from build123d import *

# Parameters (mm, degrees)
SKETCH1_W      = 31.75
SKETCH1_H      = 44.45
EXTRUDE1_DEPTH = 380


with BuildPart() as part:
    # Sketch1 → Extrude1 (new body)
    with BuildSketch(Plane(origin=(0, 0, 0), x_dir=(0, 0, -1), z_dir=(1, 0, 0))):
        with BuildLine():
            Line((-15.875, 25.4), (15.875, 25.4))
            ThreePointArc((15.875, 25.4), (18.12006403, 24.47006403), (19.05, 22.225))
            Line((19.05, 22.225), (19.05, -22.225))
            ThreePointArc((19.05, -22.225), (18.12006403, -24.47006403), (15.875, -25.4))
            Line((15.875, -25.4), (-15.875, -25.4))
            ThreePointArc((-15.875, -25.4), (-18.12006403, -24.47006403), (-19.05, -22.225))
            Line((-19.05, -22.225), (-19.05, 22.225))
            ThreePointArc((-19.05, 22.225), (-18.12006403, 24.47006403), (-15.875, 25.4))
        make_face()
        Rectangle(SKETCH1_W, SKETCH1_H, mode=Mode.SUBTRACT)
    extrude(amount=EXTRUDE1_DEPTH)


solid = part.part
Part model, mm, in its own coordinate system. A direction names the side the tool comes from. Round coordinates to 2 decimals unless told otherwise and drop trailing zeros. Loops run counter-clockwise (first coordinate to the right, second up) from the corner with the lowest first, then second, coordinate; pieces in that order, holes last. Notation, with made-up numbers: (0.25, 53) - (34.25, 53) arc R26 cw to (34.25, 68) - close; hole circle Ø4 at (77, 70.5). An arc over 180 degrees is marked (long way). Answer as a JSON object with one key per item and string values.
Item 1: Tool access for faces 1 (the face through (187, 0, -15.875)), 2 (the face through (187, 25.4, 0)): list every direction of +Z, -Z, +X, -X, +Y, -Y with a clear straight run to the whole face (end or side of a thin tool).
Output:
{"face 1": "+X, -X", "face 2": "+Z, -Z, +X, -X, +Y"}
Item 2: Band-saw the part on C-C on x = 212.5. List the corners of the cut face in (y, z) (3 decimals).
Output:
{"outline": "(-25.4, -15.875) arc R3.175 ccw to (-22.225, -19.05) - (22.225, -19.05) arc R3.175 ccw to (25.4, -15.875) - (25.4, 15.875) arc R3.175 ccw to (22.225, 19.05) - (-22.225, 19.05) arc R3.175 ccw to (-25.4, 15.875) - close; hole (-22.225, -15.875) - (22.225, -15.875) - (22.225, 15.875) - (-22.225, 15.875) - close"}
Item 3: Pull direction Z, two halves, no side cores. Call faces 3 (the face through (187, -25.4, 0)), 4 (the face through (187, 0, 19.05)), 5 (the face through (187, 22.225, 0)): pulls with the +Z half, pulls with the -Z half, needs draft (parallel to the pull), parting line crosses it, or undercut.
Output:
{"face 3": "needs draft", "face 4": "pulls with the +Z half", "face 5": "undercut"}
Item 4: Band-saw the part on A-A on z = -4. List the corners of the cut face in (x, y) (3 decimals).
Output:
{"outline": "(0, -25.4) - (380, -25.4) - (380, -22.225) - (0, -22.225) - close; (0, 22.225) - (380, 22.225) - (380, 25.4) - (0, 25.4) - close"}
Item 5: Band-saw the part on B-B on y = 16. List the corners of the cut face in (x, z) (3 decimals).
Output:
{"outline": "(0, -19.05) - (380, -19.05) - (380, -15.875) - (0, -15.875) - close; (0, 15.875) - (380, 15.875) - (380, 19.05) - (0, 19.05) - close"}
Item 6: Wall check: L1, parallel to Y at x = 114.5, z = 2.5 (3 decimals); L2, parallel to Z at x = 59.5, y = -10 (3 decimals). Give the ranges that are in metal, low to high.
Output:
{"L1": "-25.4 to -22.225, 22.225 to 25.4", "L2": "-19.05 to -15.875, 15.875 to 19.05"}
